```python
from build123d import *

# Parameters (mm, degrees)
SKETCH1_W           = 342.9
SKETCH1_H           = 225.424999902
SKETCH1_R           = 14.351
SKETCH1_R_2         = 2.9464
BOSS_EXTRUDE1_DEPTH = 6.35
SKETCH3_W           = 82.55
SKETCH3_H           = 25.4
SKETCH3_W_2         = 107.95
BOSS_EXTRUDE2_DEPTH = 6.35
SKETCH2_W           = 349.25
SKETCH2_H           = 250.824999902
CUT_EXTRUDE1_DEPTH  = 425.892825399
SKETCH4_R           = 2.54
BOSS_EXTRUDE3_DEPTH = 6.35


with BuildPart() as part:
    # Sketch1 → Boss-Extrude1 (new body)
    with BuildSketch(Plane.XY):
        with Locations((171.45, 112.712499951)):
            Rectangle(SKETCH1_W, SKETCH1_H)
        with Locations((254, 190.196999902)):
            Circle(SKETCH1_R, mode=Mode.SUBTRACT)
        with Locations((254, 21.032999902)):
            Circle(SKETCH1_R_2, mode=Mode.SUBTRACT)
        with Locations((186.255842738, 35.189941827)):
            Circle(SKETCH1_R_2, mode=Mode.SUBTRACT)
        with Locations((129.850387567, 75.291244482)):
            Circle(SKETCH1_R_2, mode=Mode.SUBTRACT)
        with Locations((63.5, 190.196999902)):
            Circle(SKETCH1_R, mode=Mode.SUBTRACT)
        with Locations((94.224517333, 134.624938265)):
            Circle(SKETCH1_R_2, mode=Mode.SUBTRACT)
        with Locations((114.3, 190.196999902)):
            Circle(SKETCH1_R, mode=Mode.SUBTRACT)
    extrude(amount=BOSS_EXTRUDE1_DEPTH)

    # Sketch3 → Boss-Extrude2 (add)
    with BuildSketch(Plane.XY.offset(6.35)):
        with Locations((41.275, 238.124999902)):
            Rectangle(SKETCH3_W, SKETCH3_H)
        with Locations((288.925, 238.124999902)):
            Rectangle(SKETCH3_W_2, SKETCH3_H)
    extrude(amount=-BOSS_EXTRUDE2_DEPTH)

    # Sketch2 → Cut-Extrude1 (cut, through all)
    with BuildSketch(Plane.XY.offset(6.35)):
        with Locations((174.625, 125.412499951)):
            Rectangle(SKETCH2_W, SKETCH2_H)
        with BuildLine():
            Line((63.5, 210.897999902), (254, 210.897999902))
            ThreePointArc((254, 210.897999902), (270.911602996, 202.135554467), (273.506313236, 183.266260769))
            ThreePointArc((273.506313236, 183.266260769), (256.315295195, 103.55517199), (260.028402179, 22.095969857))
            ThreePointArc((260.028402179, 22.095969857), (258.689264454, 17.098239828), (254, 14.911599902))
            ThreePointArc((254, 14.911599902), (151.729543137, 47.839263526), (87.882448428, 134.251217999))
            ThreePointArc((87.882448428, 134.251217999), (75.095322901, 156.248343931), (54.699389386, 171.459853539))
            ThreePointArc((54.699389386, 171.459853539), (43.295927788, 194.705532598), (63.5, 210.897999902))
        make_face(mode=Mode.SUBTRACT)
    extrude(amount=-CUT_EXTRUDE1_DEPTH, mode=Mode.SUBTRACT)

    # Sketch4 → Boss-Extrude3 (add, through all)
    with BuildSketch(Plane(origin=(0, 0, 0), x_dir=(-1, 0, 0), z_dir=(0, 0, -1))):
        with BuildLine():
            Line((14.341332207, 125.960529154), (-92.300756311, 122.533671254))
            ThreePointArc((-92.300756311, 122.533671254), (-99.071136292, 108.209082235), (-107.107329861, 94.554358196))
            Line((-107.107329861, 94.554358196), (15.054572396, 97.629850266))
            Line((15.054572396, 97.629850266), (14.341332207, 125.960529154))
        make_face()
        with Locations((0, 114.3)):
            Circle(SKETCH4_R, mode=Mode.SUBTRACT)
    extrude(amount=-BOSS_EXTRUDE3_DEPTH)


solid = part.part
```
Model file for the job. Use its own axes, mm. Give positions to 0.01 mm unless a question says otherwise; leave off trailing zeros. Order: outer loops, then holes, each group sorted by start corner. A loop starts at its lowest first (then second) coordinate and runs counter-clockwise, first axis right, second up.
1) Saw through at B-B, the plane x = 66.5. Write the cut outline in (y, z), then the cut area to 3 significant figures.
2) Pin check, flat tips, straight feed: pin 1 (1 mm diameter, centred on x = 172, z = 3.5, fed in from -Y); pin 2 (1 mm diameter, centred on x = 87.5, z = 4, fed in from -Y); pin 3 (1.5 mm diameter, centred on y = 125, z = 3.5, fed in from -X). Stop position of each tip, or through.
3) Saw through at C-C, the plane z = 5. Count the separate pieces of the cut face and the enclosed holes in it, then the cut area to 3 significant figures.
4) Mould opens along Y. For faces 1 (the cylindrical face through (256.413, 104.696, 3.219)), 2 (the cylindrical face through (270.75, 202.36, 3.22)), 3 (the cylindrical face through (171.527, 35.526, 3.219)), 4 (the flat face through (160, 114, 6.35)) say: +Y half, -Y half, draft (parallel to the pull), parting line (faces both ways), or undercut.
5) Wall check: probe 1 along Y at (x, z) = (254, 1.75); probe 2 along Y at (x, z) = (63, 4.5); probe 3 along Y at (x, z) = (105, 3.25). Give the ranges that are in metal, low to high.
6) Saw through at A-A, the plane x = 114.3. Write the cut outline in (y, z) (3 decimals).
7) Saw through at D-D, the plane y = 107. Write the cut outline in (x, z), then the cut area to 3 significant figures.
Computed:
1. outline: (95.58, 0) - (123.36, 0) - (123.36, 6.35) - (95.58, 6.35) - close; (164.25, 0) - (176.16, 0) - (176.16, 6.35) - (164.25, 6.35) - close; (204.23, 0) - (210.9, 0) - (210.9, 6.35) - (204.23, 6.35) - close
1. area: 294 mm2
2. pin 1: stops at y = 35.01
2. pin 2: stops at y = 95.04
2. pin 3: stops at x = -14.38
3. separate pieces: 1
3. enclosed holes: 8
3. area: 31,800 mm2
4. face 1: undercut
4. face 2: parting line
4. face 3: -Y half
4. face 4: draft
5. probe 1: y = 14.91 to 18.09, 23.98 to 175.85, 204.55 to 210.9
5. probe 2: y = 95.66 to 123.48, 166.77 to 175.85, 204.54 to 210.89
5. probe 3: y = 94.61 to 179.27, 201.13 to 210.9
6. outline: (84.325, 0) - (175.846, 0) - (175.846, 6.35) - (84.325, 6.35) - close; (204.548, 0) - (210.898, 0) - (210.898, 6.35) - (204.548, 6.35) - close
7. outline: (-14.82, 0) - (256.62, 0) - (256.62, 6.35) - (-14.82, 6.35) - close
7. area: 1,720 mm2
